The drawing under review shows one solid part. Ordinate dimensions are in mm from its lowest x, y, z. Round coordinates to 2 decimals unless told otherwise and drop trailing zeros. Write each loop counter-clockwise with the first axis right and the second up, starting at its lowest first coordinate (ties: lowest second). Pieces come first, ordered by that corner, then holes. Notation, with made-up numbers: (-33.5, 66.5) - (11.5, 66.5) arc R15 ccw to (11.5, 95.5) - close; hole circle Ø5 at (38, 76.5). An arc over 180 degrees is marked (long way). Answer in a Markdown table with one row per item. Add a question column.
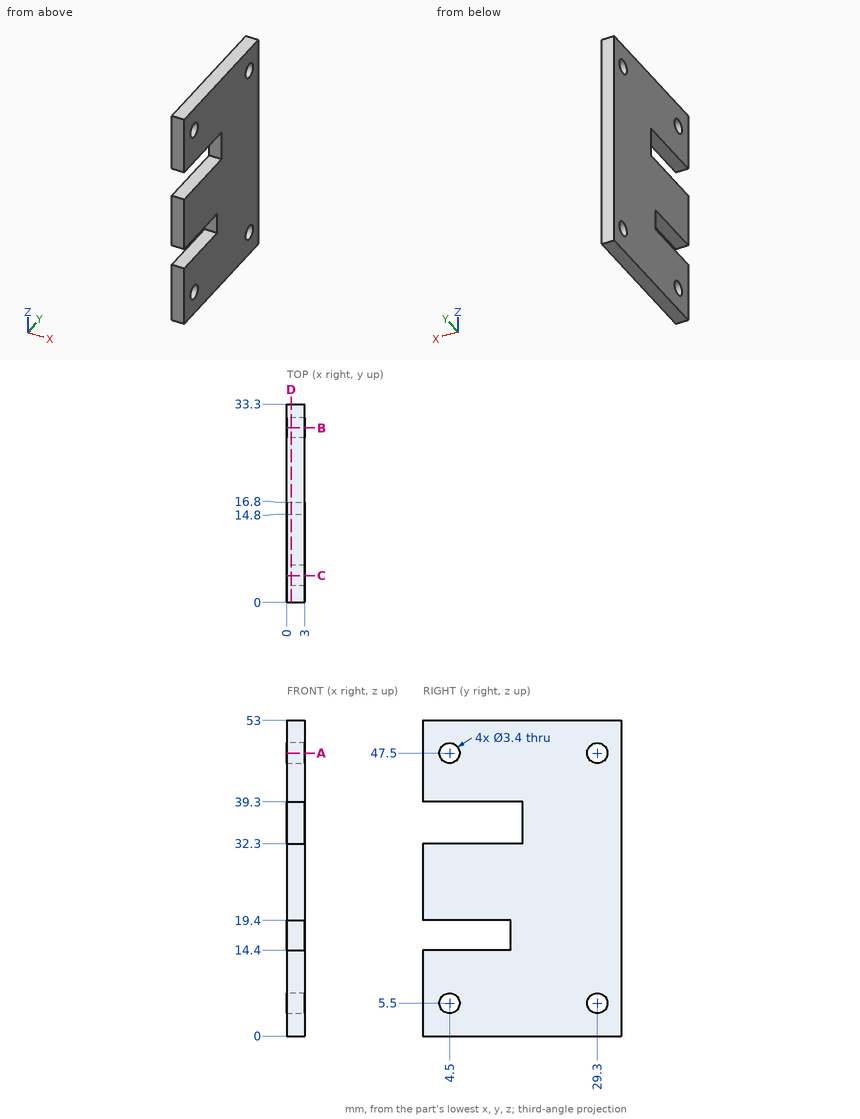
Q1. Add section C-C on y = 4.5. State the section outline as (x, z) points.
Q2. Add section D-D on x = 0.7. State the section outline as (y, z) points.
Q3. Add section A-A on z = 47.5. State the section outline as (x, y) points, then the cut area to 3 significant figures.
Q4. To check wall thickness, follow probe 1 along Y at (x, z) = (0.6, 5.5); probe 2 along Z at (x, y) = (1.35, 29.3); probe 3 along Z at (x, y) = (1.5, 4.5). State the ranges of each line that lie inside material, in increasing order.
Q5. Add section B-B on y = 29.3. State the section outline as (x, z) points.
Q6. Insertion check: pin 1 Ø1.5 at (x, z) = (2, 36.5) entering from -Y; pin 2 Ø3 at (y, z) = (4.5, 47.5) entering from -X. Each pin has a flat end and moves straight along its axis. Give the tip position at first contact, or say it passes through.
Answer sheet:
| question | item | result |
|---|---|---|
| 1 | outline | (0, 0) - (3, 0) - (3, 3.8) - (0, 3.8) - close; (0, 7.2) - (3, 7.2) - (3, 14.4) - (0, 14.4) - close; (0, 19.4) - (3, 19.4) - (3, 32.3) - (0, 32.3) - close; (0, 39.3) - (3, 39.3) - (3, 45.8) - (0, 45.8) - close; (0, 49.2) - (3, 49.2) - (3, 53) - (0, 53) - close |
| 2 | outline | (0, 0) - (33.3, 0) - (33.3, 53) - (0, 53) - (0, 39.3) - (16.8, 39.3) - (16.8, 32.3) - (0, 32.3) - (0, 19.4) - (14.8, 19.4) - (14.8, 14.4) - (0, 14.4) - close; hole circle Ø3.4 at (4.5, 5.5); hole circle Ø3.4 at (4.5, 47.5); hole circle Ø3.4 at (29.3, 5.5); hole circle Ø3.4 at (29.3, 47.5) |
| 3 | outline | (0, 0) - (3, 0) - (3, 2.8) - (0, 2.8) - close; (0, 6.2) - (3, 6.2) - (3, 27.6) - (0, 27.6) - close; (0, 31) - (3, 31) - (3, 33.3) - (0, 33.3) - close |
| 3 | area | 79.5 mm² |
| 4 | probe 1 | y = 0 to 2.8, 6.2 to 27.6, 31 to 33.3 |
| 4 | probe 2 | z = 0 to 3.8, 7.2 to 45.8, 49.2 to 53 |
| 4 | probe 3 | z = 0 to 3.8, 7.2 to 14.4, 19.4 to 32.3, 39.3 to 45.8, 49.2 to 53 |
| 5 | outline | (0, 0) - (3, 0) - (3, 3.8) - (0, 3.8) - close; (0, 7.2) - (3, 7.2) - (3, 45.8) - (0, 45.8) - close; (0, 49.2) - (3, 49.2) - (3, 53) - (0, 53) - close |
| 6 | pin 1 | stops at y = 16.8 |
| 6 | pin 2 | passes through |
